Source: CAD feature listing. Evaluate the final solid. Frame: model axes, mm. A direction names the side the tool comes from. Give positions to 0.01 mm unless a question says otherwise; leave off trailing zeros. Loops run counter-clockwise (first coordinate to the right, second up) from the corner with the lowest first, then second, coordinate; pieces in that order, holes last. Notation, with made-up numbers: (-15, 60.25) - (44, 60.25) arc R26 ccw to (44, 94.25) - close; hole circle Ø8 at (46, -1.75). An arc over 180 degrees is marked (long way). Write each question's results on one line, items separated by ' | '. Start each with the question number.
(1) Cut plane C-C on z = 21.5. Return the cut outline in (x, y), then the cut area to 3 significant figures.
(2) Material intervals for line 1 along X through (y, z) = (3, 41); line 2 along Z through (x, y) = (-23, 7); line 3 along Y through (x, z) = (-36, 28.5), sorted ascending. Write a range as [from, to].
(3) Cut plane D-D on y = 4. Return the cut outline in (x, z).
(4) Cut plane A-A on x = -19.5. Return the cut outline in (y, z).
(5) Cut plane B-B on y = 9. Return the cut outline in (x, z).
(6) Pull-direction query (X, two-part tool) for faces 1 (the flat face through (-30, 3, 30)), 2 (the flat face through (-37.85, 3.13, 30.76)), 3 (the flat face through (0, 5, 40)), 4 (the flat face through (-31, 0, 11)); classes: pulls with the +X half, pulls with the -X half, needs draft (parallel to the pull), parting line crosses it, or undercut.
(7) Reachability of faces 5 (the flat face through (-2.54, 5, -40)), 6 (the flat face through (-33, 6.35, 26)), 7 (the flat face through (-5.08, 5, 42)) from +Z, -Z, +X, -X, +Y, -Y: full face, straight path, thin tool, end or side. Return the list, or none.
(8) Contact query for flat-ended pins moving along their axis: pin 1 (4 mm diameter, centred on x = -18.5, y = 7, fed in from +Z); pin 2 (3 mm diameter, centred on y = 7.5, z = 39, fed in from -X); pin 3 (3 mm diameter, centred on y = 7, z = -38, fed in from +X). Output: stop coordinate, or through.
from build123d import *

# Parameters (mm, degrees)
BOSS_EXTRUDE1_DEPTH = 10.16
SKETCH3_W           = 10.16
SKETCH3_H           = 5.08
BOSS_EXTRUDE2_DEPTH = 16.51
SKETCH4_W           = 10.16
SKETCH4_H           = 5.08
BOSS_EXTRUDE3_DEPTH = 16.51
BOSS_EXTRUDE5_DEPTH = 6.35


with BuildPart() as part:
    # Sketch1 → Boss-Extrude1 (new body)
    with BuildSketch(Plane(origin=(0, 0, 0), x_dir=(1, 0, 0), z_dir=(0, 1, 0))):
        with BuildLine():
            Line((0, -32.004), (0, -35.179))
            ThreePointArc((0, -35.179), (-35.156038364, -1.270829481), (-2.54, 35.087183429))
            Line((-2.54, 35.087183429), (-2.54, 31.903047127))
            ThreePointArc((-2.54, 31.903047127), (-31.978751823, -1.271002703), (0, -32.004))
        make_face()
    extrude(amount=BOSS_EXTRUDE1_DEPTH)

    # Sketch3 → Boss-Extrude2 (add)
    with BuildSketch(Plane(origin=(0, 0, 32.004), x_dir=(0, -1, 0), z_dir=(0, 0, -1))):
        with Locations((-5.08, 2.54)):
            Rectangle(SKETCH3_W, SKETCH3_H)
    extrude(amount=-BOSS_EXTRUDE2_DEPTH)

    # Sketch4 → Boss-Extrude3 (add)
    with BuildSketch(Plane(origin=(0, 0, -32.004), x_dir=(0, -1, 0), z_dir=(0, 0, 1))):
        with Locations((-5.08, -5.08)):
            Rectangle(SKETCH4_W, SKETCH4_H)
    extrude(amount=-BOSS_EXTRUDE3_DEPTH)

    # Sketch6 → Boss-Extrude5 (add)
    with BuildSketch(Plane.XZ):
        Polygon((-22.630245425, 22.630245425), (-34.304578382, 34.304578382), (-41.488783279, 27.120373486), (-29.814450322, 15.446040528), align=None)
    extrude(amount=-BOSS_EXTRUDE5_DEPTH)


solid = part.part
Ans:
1) outline: (-35.87, 0) - (-23.71, 0) - (-23.71, 10.16) - (-27.84, 10.16) - (-27.84, 6.35) - (-35.87, 6.35) - close | area: 93.0 mm^2
2) line 1: [-5.08, 0] | line 2: [-26.62, -22.25], [22.25, 26.62] | line 3: [0, 6.35]
3) outline: (-41.49, 27.12) - (-31, 16.63) arc R35.18 ccw to (-7.62, -34.34) - (-7.62, -48.51) - (-2.54, -48.51) - (-2.54, -31.9) arc R32 cw to (0, 32) - (0, 48.51) - (-5.08, 48.51) - (-5.08, 34.81) arc R35.18 ccw to (-24.88, 24.88) - (-34.3, 34.3) - close
4) outline: (0, -29.28) - (10.16, -29.28) - (10.16, -25.38) - (0, -25.38) - close; (0, 25.38) - (10.16, 25.38) - (10.16, 29.28) - (0, 29.28) - close
5) outline: (-7.62, -48.51) - (-2.54, -48.51) - (-2.54, -31.9) arc R32 cw to (0, 32) - (0, 48.51) - (-5.08, 48.51) - (-5.08, 34.81) arc R35.18 ccw to (-7.62, -34.34) - close
6) face 1: undercut | face 2: pulls with the -X half | face 3: pulls with the +X half | face 4: needs draft
7) face 5: -Z, +X, +Y, -Y | face 6: +Z, -X, +Y | face 7: +Z, -X, +Y, -Y
8) pin 1: z = 31.07 | pin 2: x = -5.08 | pin 3: x = -2.54
